Check sheet for the modelled part. Datum: model origin and axes. Units: mm. A direction names the side the tool comes from. Round coordinates to 2 decimals unless told otherwise and drop trailing zeros. Order: outer loops, then holes, each group sorted by start corner. A loop starts at its lowest first (then second) coordinate and runs counter-clockwise, first axis right, second up.
Q1. Scan lines: probe 1 along X at (y, z) = (1.05, -3.5); probe 2 along X at (y, z) = (9.5, 0.75); probe 3 along Y at (x, z) = (0, -12.3). Record each from-to range of solid material in increasing order.
Q2. Cross-section at C-C on z = 5.5. Record the cut outline in (x, y), then the cut area to 4 significant figures.
Q3. Depth check by flat-ended pin: P1, Ø1, axis at x = -7, y = 3, coming from the +Z side; P2, Ø11, axis at x = -4, z = -5, coming from the +Y side; P3, Ø3, axis at x = 0, z = 5.5, coming from the -Y side. Enter the tip coordinate at first touch or a pass-through.
Q4. Cross-section at B-B on y = 9.5. Record the cut outline in (x, z), then the cut area to 3 significant figures.
Q5. Mould release check, pull along Z, two halves, no side actions. Record for faces 3 (the flat face through (0, 17, -12)), 4 (the flat face through (12.014, 9.605, 0.832)), 5 (the cylindrical face through (-0.61, 1.01, 6.98)): +Z half, -Z half, draft (parallel to the pull), parting line (faces both ways), or undercut.
Q6. Cross-section at A-A on x = 0. Record the cut outline in (y, z).
Q7. Set-up check for faces 1 (the flat face through (-0.2, 7.7, -11)), 2 (the flat face through (0, 6, -13)): record each of +Z, -Z, +X, -X, +Y, -Y from which the full face is reachable in a straight line by a thin tool's end or side.
Q8. Cross-section at D-D on y = 15. Record the cut outline in (x, z).
from build123d import *

# Parameters (mm, degrees)
SKETCH_1_W          = 26
SKETCH_1_H          = 26
EXTRUDE_1_DEPTH     = 17
CUT_EXTRUDE_1_DEPTH = 34.674916481
SHELL_START         = -11
SHELL_2_DEPTH       = 22
SKETCH_3_R          = 1.6
CUT_EXTRUDE_2_DEPTH = 24.727621035
SKETCH_4_R          = 1.6
CUT_EXTRUDE_3_DEPTH = 33.155870382


# Read off the part's stored shape, not the designer's step: ｼｪﾙ2
with BuildPart() as part:
    # ｽｹｯﾁ1 → ﾎﾞｽ - 押し出し1 (new body)
    with BuildSketch(Plane(origin=(0, 0, 0), x_dir=(1, 0, 0), z_dir=(0, 1, 0))):
        Rectangle(SKETCH_1_W, SKETCH_1_H)
    extrude(amount=EXTRUDE_1_DEPTH)

    # ｽｹｯﾁ2 → ｶｯﾄ - 押し出し1 (cut, through all)
    with BuildSketch(Plane(origin=(13, 0, 0), x_dir=(0, 0, -1), z_dir=(1, 0, 0))):
        Polygon((11, 17), (-13, 2), (-13, 17), align=None)
    extrude(amount=-CUT_EXTRUDE_1_DEPTH, mode=Mode.SUBTRACT)

    # ｼｪﾙ2 outline → ｼｪﾙ2 (cut)
    with BuildSketch(Plane.YZ.offset(SHELL_START)):
        Polygon((2, -11), (17, -11), (2, 13), align=None)
    extrude(amount=SHELL_2_DEPTH, mode=Mode.SUBTRACT)

    # ｽｹｯﾁ3 → ｶｯﾄ - 押し出し2 (cut, through all)
    with BuildSketch(Plane(origin=(0, 2, 0), x_dir=(1, 0, 0), z_dir=(0, 1, 0))):
        with Locations(Location((0, 3.5, 0), (0, 0, 270))):
            Circle(SKETCH_3_R)
        with Locations(Location((0, -5.5, 0), (0, 0, 270))):
            Circle(SKETCH_3_R)
    extrude(amount=-CUT_EXTRUDE_2_DEPTH, mode=Mode.SUBTRACT)

    # ｽｹｯﾁ4 → ｶｯﾄ - 押し出し3 (cut, through all)
    with BuildSketch(Plane.XY.offset(-11)):
        with Locations((0, 9.5)):
            Circle(SKETCH_4_R)
    extrude(amount=-CUT_EXTRUDE_3_DEPTH, mode=Mode.SUBTRACT)


solid = part.part
Results found:
1. probe 1: x = -13 to -1.6, 1.6 to 13
1. probe 2: x = -13 to -11, 11 to 13
1. probe 3: y = 0 to 7.9, 11.1 to 17
2. outline: (-13, 0) - (-1.6, 0) - (-1.6, 2) - (-11, 2) - (-11, 6.69) - (-13, 6.69) - close; (1.6, 0) - (13, 0) - (13, 6.69) - (11, 6.69) - (11, 2) - (1.6, 2) - close
2. area: 64.35 mm2
3. P1: stops at z = -11
3. P2: stops at y = 2
3. P3: passes through
4. outline: (-13, -13) - (-1.6, -13) - (-1.6, -11) - (-11, -11) - (-11, 1) - (-13, 1) - close; (1.6, -13) - (13, -13) - (13, 1) - (11, 1) - (11, -11) - (1.6, -11) - close
4. area: 93.6 mm2
5. face 3: draft
5. face 4: +Z half
5. face 5: undercut
6. outline: (0, -13) - (7.9, -13) - (7.9, -11) - (2, -11) - (2, -5.1) - (0, -5.1) - close; (0, -1.9) - (2, -1.9) - (2, 3.9) - (0, 3.9) - close; (0, 7.1) - (2, 7.1) - (2, 13) - (0, 13) - close; (11.1, -13) - (17, -13) - (17, -11) - (11.1, -11) - close
7. face 1: +Z, +Y
7. face 2: -Z, +X, -X, +Y, -Y
8. outline: (-13, -13) - (13, -13) - (13, -7.8) - (11, -7.8) - (11, -11) - (-11, -11) - (-11, -7.8) - (-13, -7.8) - close
